Design review of the part built by this model. Coordinates are the model's own, in mm. A direction names the side the tool comes from. Coordinates: 2 decimals unless noted, no trailing zeros. Loops run counter-clockwise (first coordinate to the right, second up) from the corner with the lowest first, then second, coordinate; pieces in that order, holes last.
Q1. For P1, Ø10, axis at y = 18.5, z = -62, coming from the -X side; P2, Ø6, axis at y = 18.5, z = 30, coming from the -X side; P3, Ø4, axis at x = -116.5, z = 37.5, coming from the +Y side, all flat-tipped, find the tip position at first contact; note any pin that passes through.
Q2. Machinability: for faces 1 (the face through (-1, 1, -75)), 2 (the face through (227, 28, 1)), which of the approach directions +Z, -Z, +X, -X, +Y, -Y give a long, thin tool a straight path to every point of the face, cutting with its end or side? Answer none if there is none.
Q3. Draft analysis for pull direction Y (two halves, no side actions). For faces 3 (the face through (-3, 3, -1)), 4 (the face through (228.48, 17.04, 58.49)), 5 (the face through (-3, 0, -1)), 6 (the face through (-228.479, 18.667, -26.204)), state which applies: released by +Y, released by -Y, zero draft, split by the parting line, or undercut.
Q4. Add section A-A on y = 39.5. Give the boundary of the cut face in (x, z).
Q5. Add section C-C on x = 78. Give the boundary of the cut face in (y, z), and give its area (3 significant figures).
Q6. Add section B-B on z = 48.5. Give the boundary of the cut face in (x, y), and give its area (3 significant figures).
Q7. Wall thickness on probe 1 along Z at (x, y) = (229.3, 18.5); probe 2 along X at (y, z) = (34, 30); probe 3 along Y at (x, z) = (229, -30): over which ranges is each line inside the solid? List them lowest first.
```python
from build123d import *

# Parameters (mm, degrees)
SKETCH1_W               = 460
SKETCH1_H               = 150
BOSS_EXTRUDE1_DEPTH     = 3
SKETCH2_W               = 3
SKETCH2_H               = 150
BOSS_EXTRUDE2_DEPTH     = 50
SKETCH4_R               = 3.8
CUT_EXTRUDE1_DEPTH      = 458
CUT_EXTRUDE1_DEPTH_BACK = 4
CUT_EXTRUDE2_DEPTH      = 10


with BuildPart() as part:
    # Sketch1 → Boss-Extrude1 (new body)
    with BuildSketch(Plane(origin=(0, 0, 0), x_dir=(1, 0, 0), z_dir=(0, 1, 0))):
        Rectangle(SKETCH1_W, SKETCH1_H)
    extrude(amount=BOSS_EXTRUDE1_DEPTH)

    # Sketch2 → Boss-Extrude2 (add)
    with BuildSketch(Plane(origin=(0, 3, 0), x_dir=(1, 0, 0), z_dir=(0, 1, 0))):
        with Locations((-228.5, 0)):
            Rectangle(SKETCH2_W, SKETCH2_H)
        with Locations((228.5, 0)):
            Rectangle(SKETCH2_W, SKETCH2_H)
    extrude(amount=BOSS_EXTRUDE2_DEPTH)

    # Sketch4 → Cut-Extrude1 (cut, two sides)
    with BuildSketch(Plane(origin=(-227, 0, 0), x_dir=(0, 0, -1), z_dir=(1, 0, 0))) as cut_extrude1_sk:
        with Locations((62, 18.5)):
            Circle(SKETCH4_R)
        with Locations((30, 18.5)):
            Circle(SKETCH4_R)
        with Locations((-62, 18.5)):
            Circle(SKETCH4_R)
        with Locations((-30, 18.5)):
            Circle(SKETCH4_R)
    extrude(amount=CUT_EXTRUDE1_DEPTH, mode=Mode.SUBTRACT)
    extrude(cut_extrude1_sk.sketch, amount=-CUT_EXTRUDE1_DEPTH_BACK, mode=Mode.SUBTRACT)

    # Sketch5 → Cut-Extrude2 (cut)
    with BuildSketch(Plane(origin=(0, 3, 0), x_dir=(1, 0, 0), z_dir=(0, 1, 0))):
        with BuildLine():
            ThreePointArc((174.5, -8), (171.5, -11), (174.5, -14))
            Line((174.5, -14), (174.5, -8))
        make_face()
        with BuildLine():
            Line((174.5, -8), (174.5, -14))
            ThreePointArc((174.5, -14), (176.621320344, -13.121320344), (177.5, -11))
            ThreePointArc((177.5, -11), (176.621320344, -8.878679656), (174.5, -8))
        make_face()
        with BuildLine():
            Line((174.5, -14), (204.5, -14))
            ThreePointArc((204.5, -14), (201.5, -11), (204.5, -8))
            Line((204.5, -8), (174.5, -8))
            ThreePointArc((174.5, -8), (176.621320344, -8.878679656), (177.5, -11))
            ThreePointArc((177.5, -11), (176.621320344, -13.121320344), (174.5, -14))
        make_face()
        with BuildLine():
            ThreePointArc((204.5, -8), (201.5, -11), (204.5, -14))
            Line((204.5, -14), (204.5, -8))
        make_face()
        with BuildLine():
            Line((204.5, -8), (204.5, -14))
            ThreePointArc((204.5, -14), (206.621320344, -13.121320344), (207.5, -11))
            ThreePointArc((207.5, -11), (206.621320344, -8.878679656), (204.5, -8))
        make_face()
        with BuildLine():
            ThreePointArc((204.5, 14), (201.5, 11), (204.5, 8))
            Line((204.5, 8), (204.5, 14))
        make_face()
        with BuildLine():
            Line((204.5, 14), (204.5, 8))
            ThreePointArc((204.5, 8), (206.621320344, 8.878679656), (207.5, 11))
            ThreePointArc((207.5, 11), (206.621320344, 13.121320344), (204.5, 14))
        make_face()
        with BuildLine():
            ThreePointArc((177.5, 11), (176.621320344, 8.878679656), (174.5, 8))
            Line((174.5, 8), (204.5, 8))
            ThreePointArc((204.5, 8), (201.5, 11), (204.5, 14))
            Line((204.5, 14), (174.5, 14))
            ThreePointArc((174.5, 14), (176.621320344, 13.121320344), (177.5, 11))
        make_face()
        with BuildLine():
            ThreePointArc((174.5, 14), (171.5, 11), (174.5, 8))
            Line((174.5, 8), (174.5, 14))
        make_face()
        with BuildLine():
            Line((174.5, 14), (174.5, 8))
            ThreePointArc((174.5, 8), (176.621320344, 8.878679656), (177.5, 11))
            ThreePointArc((177.5, 11), (176.621320344, 13.121320344), (174.5, 14))
        make_face()
    extrude(amount=-CUT_EXTRUDE2_DEPTH, mode=Mode.SUBTRACT)


solid = part.part
```
Entries:
1. P1: stops at x = -230
1. P2: passes through
1. P3: stops at y = 3
2. face 1: -Z, +X, -X, +Y, -Y
2. face 2: +Z, -Z, +Y
3. face 3: released by +Y
3. face 4: undercut
3. face 5: released by -Y
3. face 6: undercut
4. outline: (-230, -75) - (-227, -75) - (-227, 75) - (-230, 75) - close; (227, -75) - (230, -75) - (230, 75) - (227, 75) - close
5. outline: (0, -75) - (3, -75) - (3, 75) - (0, 75) - close
5. area: 450 mm2
6. outline: (-230, 0) - (230, 0) - (230, 53) - (227, 53) - (227, 3) - (-227, 3) - (-227, 53) - (-230, 53) - close
6. area: 1,680 mm2
7. probe 1: z = -75 to -65.8, -58.2 to -33.8, -26.2 to 26.2, 33.8 to 58.2, 65.8 to 75
7. probe 2: x = -230 to -227, 227 to 230
7. probe 3: y = 0 to 14.7, 22.3 to 53
